Part model, mm, in its own coordinate system. Face numbers are marked on the shaded views. Give positions to 0.01 mm unless a question says otherwise; leave off trailing zeros. Order: outer loops, then holes, each group sorted by start corner. A loop starts at its lowest first (then second) coordinate and runs counter-clockwise, first axis right, second up. Notation, with made-up numbers: M 64.25,49.5 L 79.25,49.5 A10 ccw 79.25,63.5 Z; hole C -7.5,-13.75 d2. An arc over 180 degrees is marked long. One line per question, with ' | ' between items.
```python
from build123d import *

# Parameters (mm, degrees)
SKETCH1_W           = 15
SKETCH1_H           = 14
SKETCH1_R           = 3.25
BOSS_EXTRUDE1_DEPTH = 2
SKETCH2_R           = 5
SKETCH2_R_2         = 3.5
BOSS_EXTRUDE2_DEPTH = 22.5
BOSS_EXTRUDE3_DEPTH = 4
CHAMFER1_SIZE       = 3
FILLET1_R           = 2


with BuildPart() as part:
    # Sketch1 → Boss-Extrude1 (new body)
    with BuildSketch(Plane.XY):
        Rectangle(SKETCH1_W, SKETCH1_H)
        Circle(SKETCH1_R, mode=Mode.SUBTRACT)
    extrude(amount=BOSS_EXTRUDE1_DEPTH)



with BuildPart() as body_2:
    # Sketch2 → Boss-Extrude2 (new body)
    with BuildSketch(Plane(origin=(7.5, 0, 0), x_dir=(0, 0, -1), z_dir=(1, 0, 0))):
        with Locations(Location((-6, 0, 0), (0, 0, 180))):
            Circle(SKETCH2_R)
        with Locations(Location((-6, 0, 0), (0, 0, 180))):
            Circle(SKETCH2_R_2, mode=Mode.SUBTRACT)
    extrude(amount=BOSS_EXTRUDE2_DEPTH)


with BuildPart() as part_1:
    add(part.part)

    add(body_2.part)  # Boss-Extrude3 merges body 2
    # Sketch3 → Boss-Extrude3 (add)
    with BuildSketch(Plane(origin=(7.5, 0, 0), x_dir=(0, 0, -1), z_dir=(1, 0, 0))):
        with BuildLine():
            Line((-7.867068249, 4.638324714), (-2, 7))
            Line((-2, 7), (0, 7))
            Line((0, 7), (0, -7))
            Line((0, -7), (-2, -7))
            Line((-2, -7), (-7.867068249, -4.638324714))
            ThreePointArc((-7.867068249, -4.638324714), (-11, 0), (-7.867068249, 4.638324714))
        make_face()
    extrude(amount=BOSS_EXTRUDE3_DEPTH)

    # Chamfer1
    chamfer1_edges = [part_1.edges().sort_by_distance(p)[0] for p in [
        (7.5, -2.798629911, 10.143388785),
        (7.5, -5.819162357, 4.933534125),
        (7.5, 5.819162357, 4.933534125),
    ]]
    chamfer(chamfer1_edges, length=CHAMFER1_SIZE)

    # Fillet1
    fillet1_edges = [part_1.edges().sort_by_distance(p)[0] for p in [
        (-7.5, 7, 1),
        (-7.5, -7, 1),
    ]]
    fillet(fillet1_edges, radius=FILLET1_R)


solid = part_1.part
```
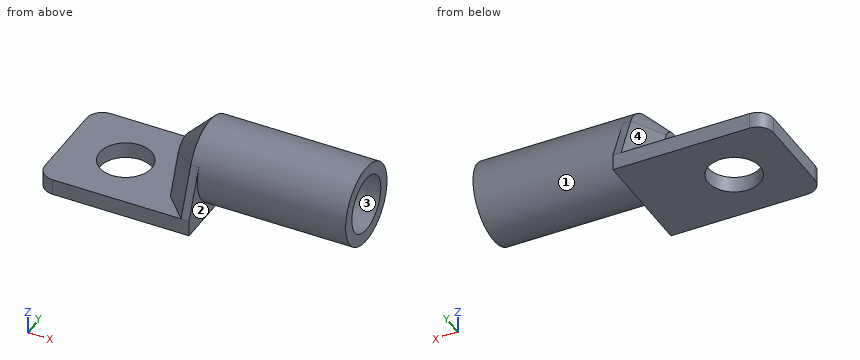
1. Slice it at D-D on x = 26. Give the cut face in (y, z).
Worked out:
outline: C 0,6 d10; hole C 0,6 d7
2. Drop flat-ended pins along their axis: pin 1 (6 mm diameter, centred on y = 4.5, z = 5.5, fed in from -X); pin 2 (2 mm diameter, centred on y = 0.5, z = 4.5, fed in from +X); pin 3 (3 mm diameter, centred on x = 9.5, z = 6, fed in from +Y); pin 4 (5 mm diameter, centred on y = 1, z = 4, fed in from -X). Give the stop position or say it passes through.
Worked out:
pin 1: stops at x = 7.5 | pin 2: stops at x = 11.5 | pin 3: stops at y = 5.84 | pin 4: stops at x = -7.5
3. Slice it at B-B on x = 0. Give the cut face in (y, z).
Worked out:
outline: M -7,0 L -3.25,0 L -3.25,2 L -7,2 Z; M 3.25,0 L 7,0 L 7,2 L 3.25,2 Z
4. Probe L1, parallel to Y at x = 0, z = 1.3; L2, parallel to Z at x = 6, y = 3.25; L3, parallel to Y at x = 18, z = 6. List the from-to ranges inside material, lowest first. Write a range as from..to.
Worked out:
L1: y = -7..-3.25, 3.25..7 | L2: z = 0..2 | L3: y = -5..-3.5, 3.5..5
5. Slice it at C-C on z = 1.5. Give the cut face in (x, y), then the cut area to 3 significant figures.
Worked out:
outline: M -7.5,-5 A2 ccw -5.5,-7 L 11.5,-7 L 11.5,-2.18 L 30,-2.18 L 30,2.18 L 11.5,2.18 L 11.5,7 L -5.5,7 A2 ccw -7.5,5 Z; hole C 0,0 d6.5 | area: 312 mm2
6. Mould opens along Z. For the marked faces 1, 2, 3 and 4 say: released by +Z, released by -Z, zero draft, split by the parting line, or undercut.
Worked out:
face 1: split by the parting line | face 2: zero draft | face 3: undercut | face 4: released by +Z
7. Slice it at A-A on y = 0. Give the cut face in (x, z), then the cut area to 3 significant figures.
Worked out:
outline: M -7.5,0 L -3.25,0 L -3.25,2 L -7.5,2 Z; M 3.25,0 L 11.5,0 L 11.5,1 L 30,1 L 30,2.5 L 11.5,2.5 L 11.5,9.5 L 30,9.5 L 30,11 L 10.5,11 L 7.5,8 L 7.5,2 L 3.25,2 Z | area: 112 mm2
